Design review of the part built by this model. Coordinates are the model's own, in mm. A direction names the side the tool comes from. Give positions to 0.01 mm unless a question says otherwise; leave off trailing zeros. Write each loop counter-clockwise with the first axis right and the second up, starting at its lowest first coordinate (ties: lowest second). Pieces come first, ordered by that corner, then holes. Notation, with made-up numbers: M -14,59.5 L 3,59.5 A19 ccw 3,90.5 Z; hole C -34,22.25 d1. An arc over 180 degrees is marked long. Use one line per item in the form item = value. Start each with the question number.
from build123d import *

# Parameters (mm, degrees)
PAD_DEPTH    = 5.5
SKETCH001_W  = 89.8
SKETCH001_H  = 9.3
POCKET_DEPTH = 3.75
SKETCH002_R  = 3.1
PAD001_DEPTH = 4.3


with BuildPart() as part:
    # Sketch → Pad (new body)
    with BuildSketch(Plane.XY):
        Polygon((0, 0), (97.7, 0), (97.7, 23.8), (93.4, 23.8), (93.4, 15.6), (4.3, 15.6), (4.3, 23.8), (0, 23.8), align=None)
    extrude(amount=PAD_DEPTH)

    # Sketch001 (on Face10 of Pad) → Pocket (cut)
    with BuildSketch(Plane.XY.offset(5.5)):
        with Locations((48.9, 8.15)):
            Rectangle(SKETCH001_W, SKETCH001_H)
    extrude(amount=-POCKET_DEPTH, mode=Mode.SUBTRACT)

    # Sketch002 (on Face2 of Pocket) → Pad001 (join)
    with BuildSketch(Plane(origin=(0, 0, 0), x_dir=(0, -1, 0), z_dir=(-1, 0, 0))):
        with Locations((-20.69, 3.1)):
            Circle(SKETCH002_R)
    extrude(amount=-PAD001_DEPTH)


solid = part.part
1. We need section C-C (x = 62). State the section outline as (y, z) points.
2. Draft analysis for pull direction Y (two halves, no side actions). For faces 1 (the flat face through (0, 12, 3)), 2 (the flat face through (48, 12.8, 4)), 3 (the flat face through (48, 0, 3)), 4 (the flat face through (4, 8, 4)), state which applies: pulls with the +Y half, pulls with the -Y half, needs draft (parallel to the pull), parting line crosses it, or undercut.
3. We need section A-A (y = 20.25). State the section outline as (x, z) points, and give its area (3 significant figures).
4. To check wall thickness, follow L1, parallel to Y at x = 19, z = 3.5; L2, parallel to X at y = 7.25, z = 2; L3, parallel to X at y = 22.5, z = 5. State the ranges of each line that lie inside material, in increasing order.
5. Clearance check with flat-ended pins moving along their axes: pin 1 Ø1.3 at (x, y) = (1.5, 23) entering from +Z; pin 2 Ø4.5 at (x, y) = (71, 9.5) entering from +Z; pin 3 Ø3 at (x, z) = (82.5, 2.5) entering from +Y. State where each tip first meets the part, or that it passes through.
6. We need section B-B (z = 3). State the section outline as (x, y) points.
7. We need section D-D (y = 4.5). State the section outline as (x, z) points.
8. For faces 5 (the flat face through (93.8, 8, 4)), 6 (the flat face through (49, 15.6, 3)), 7 (the flat face through (96, 23.8, 3)), list the 3-axis set-ups (+Z, -Z, +X, -X, +Y, -Y) from which the entire face can be reached by the end or side of a thin tool; tool diameter is ignored.
Answer block:
q1.outline = M 0,0 L 15.6,0 L 15.6,5.5 L 12.8,5.5 L 12.8,1.75 L 3.5,1.75 L 3.5,5.5 L 0,5.5 Z
q2.face_1 = needs draft
q2.face_2 = undercut
q2.face_3 = pulls with the -Y half
q2.face_4 = undercut
q3.outline = M 0,0 L 4.3,0 L 4.3,6.17 L 0,6.17 Z; M 93.4,0 L 97.7,0 L 97.7,5.5 L 93.4,5.5 Z
q3.area = 50.2 mm^2
q4.L1 = 0 to 3.5, 12.8 to 15.6
q4.L2 = 0 to 4, 93.8 to 97.7
q4.L3 = 0 to 4.3, 93.4 to 97.7
q5.pin_1 = 5.72
q5.pin_2 = 1.75
q5.pin_3 = 15.6
q6.outline = M 0,0 L 97.7,0 L 97.7,23.8 L 93.4,23.8 L 93.4,15.6 L 4.3,15.6 L 4.3,23.8 L 0,23.8 Z; hole M 4,3.5 L 93.8,3.5 L 93.8,12.8 L 4,12.8 Z
q7.outline = M 0,0 L 97.7,0 L 97.7,5.5 L 93.8,5.5 L 93.8,1.75 L 4,1.75 L 4,5.5 L 0,5.5 Z
q8.face_5 = +Z
q8.face_6 = +Z, -Z, +Y
q8.face_7 = +Z, -Z, +X, -X, +Y
